Part model, mm, in its own coordinate system. A direction names the side the tool comes from. Give positions to 0.01 mm unless a question says otherwise; leave off trailing zeros. Order: outer loops, then holes, each group sorted by start corner. A loop starts at its lowest first (then second) coordinate and runs counter-clockwise, first axis right, second up.
1. Slice it at D-D on z = 10. List the corners of the cut face in (x, y).
2. Slice it at C-C on x = 0. Give the number of separate pieces and of enclosed holes in the cut face, and give its area (3 significant figures).
3. Drop flat-ended pins along their axis: pin 1 Ø10 at (x, z) = (6.5, -14.5) entering from -Y; pin 2 Ø12 at (x, y) = (42.5, 106.5) entering from -Z; pin 3 Ø1 at (x, y) = (24.5, 27) entering from +Z; pin 4 Ø1 at (x, z) = (-0.5, 14.5) entering from -Y. Give the stop position or say it passes through.
4. Which spindle directions (+Z, -Z, +X, -X, +Y, -Y) get a long thin tool onto all of the face, cutting with end or side? Do faces 4 (the flat face through (55, 110, 6)), 5 (the flat face through (-12, 12, 8)), 6 (the flat face through (0, 33, -40)), 7 (the flat face through (-5.9, 121.5, -43)), 8 (the flat face through (-5.9, 121.5, 3)). Say none if no direction does.
5. Probe line 1 (Y direction, x = 0, z = -32.5); line 2 (Y direction, x = 0, z = -25); line 3 (Y direction, x = 0, z = -17). List the from-to ranges inside material, lowest first.
6. Mould opens along X. For faces 1 (the flat face through (55, 110, -24)), 2 (the flat face through (-12, 12, -26)), 3 (the flat face through (25, 43, -9)) say: +X half, -X half, draft (parallel to the pull), parting line (faces both ways), or undercut.
7. Slice it at B-B on z = -20. List the corners of the cut face in (x, y), and give its area (3 significant figures).
8. Slice it at A-A on y = 0. List the corners of the cut face in (x, z).
from build123d import *

# Parameters (mm, degrees)
BOSS_EXTRUDE1_DEPTH      = 3
BOSS_EXTRUDE1_DEPTH_BACK = 43
SKETCH1_R                = 25
SKETCH1_R_2              = 12.5
BOSS_EXTRUDE2_DEPTH      = 18
SKETCH2_R                = 28
SKETCH2_R_2              = 16
BOSS_EXTRUDE3_DEPTH      = 35
BOSS_EXTRUDE4_DEPTH      = 31
CUT_EXTRUDE1_DEPTH       = 152.558569537
CUT_EXTRUDE1_DEPTH_BACK  = 152.558569537
SKETCH3_W                = 34
SKETCH3_H                = 83.380174096
SKETCH4_R                = 18
SKETCH4_R_2              = 7.5
BOSS_EXTRUDE5_DEPTH      = 24
BOSS_EXTRUDE6_DEPTH      = 21
BOSS_EXTRUDE7_DEPTH      = 9


with BuildPart() as part:
    # Sketch1 → Boss-Extrude1 (new, two sides: drawn at the far end of the back side and taken through both)
    with BuildSketch(Plane.XY.offset(-BOSS_EXTRUDE1_DEPTH_BACK)):
        with Locations((0, 110)):
            Circle(SKETCH1_R)
        with Locations((0, 110)):
            Circle(SKETCH1_R_2, mode=Mode.SUBTRACT)
    extrude(amount=BOSS_EXTRUDE1_DEPTH + BOSS_EXTRUDE1_DEPTH_BACK)

    # Sketch1_3 → Boss-Extrude2 (add)
    with BuildSketch(Plane.XY):
        with BuildLine():
            ThreePointArc((25, 110), (0, 85), (-25, 110))
            Line((-25, 110), (-25, 40))
            Line((-25, 40), (25, 40))
            Line((25, 40), (25, 110))
        make_face()
    extrude(amount=-BOSS_EXTRUDE2_DEPTH)



with BuildPart() as body_2:
    # Sketch2 → Boss-Extrude3 (new, symmetric)
    with BuildSketch(Plane.XY.offset(-9)):
        Circle(SKETCH2_R)
        Circle(SKETCH2_R_2, mode=Mode.SUBTRACT)
    extrude(amount=BOSS_EXTRUDE3_DEPTH, both=True)


with BuildPart() as part_1:
    add(part.part)

    add(body_2.part)  # Boss-Extrude4 merges body 2
    # Sketch2_3 → Boss-Extrude4 (add, symmetric)
    with BuildSketch(Plane.XY.offset(-9)):
        with BuildLine():
            Line((25, 40), (-25, 40))
            Line((-25, 40), (-25, 12.609520213))
            ThreePointArc((-25, 12.609520213), (0, 28), (25, 12.609520213))
            Line((25, 12.609520213), (25, 40))
        make_face()
    extrude(amount=BOSS_EXTRUDE4_DEPTH, both=True)

    # Sketch3 → Cut-Extrude1 (cut, two sides: drawn at the far end of the back side and taken through both)
    with BuildSketch(Plane.ZY.offset(25).offset(-CUT_EXTRUDE1_DEPTH_BACK)):
        with Locations((-9, -13.690087048)):
            Rectangle(SKETCH3_W, SKETCH3_H)
    extrude(amount=CUT_EXTRUDE1_DEPTH + CUT_EXTRUDE1_DEPTH_BACK, mode=Mode.SUBTRACT)



with BuildPart() as body_2_2:
    # Sketch4 → Boss-Extrude5 (new, symmetric)
    with BuildSketch(Plane.XY.offset(-9)):
        with Locations((85, 110)):
            Circle(SKETCH4_R)
        with Locations((85, 110)):
            Circle(SKETCH4_R_2, mode=Mode.SUBTRACT)
    extrude(amount=BOSS_EXTRUDE5_DEPTH, both=True)

    # Sketch4_3 → Boss-Extrude6 (add, symmetric)
    with BuildSketch(Plane.XY.offset(-9)):
        with BuildLine():
            Line((55, 110), (67, 110))
            ThreePointArc((67, 110), (72.272077939, 122.727922061), (85, 128))
            Line((85, 128), (55, 128))
            Line((55, 128), (55, 110))
        make_face()
        with BuildLine():
            ThreePointArc((85, 92), (72.272077939, 97.272077939), (67, 110))
            Line((67, 110), (55, 110))
            Line((55, 110), (55, 92))
            Line((55, 92), (85, 92))
        make_face()
    extrude(amount=BOSS_EXTRUDE6_DEPTH, both=True)


with BuildPart() as part_2:
    add(part_1.part)

    add(body_2_2.part)  # Boss-Extrude7 merges body 2 2
    # Sketch4_4 → Boss-Extrude7 (add, symmetric)
    with BuildSketch(Plane.XY.offset(-9)):
        with BuildLine():
            Line((25, 110), (55, 110))
            Line((55, 110), (55, 128))
            Line((55, 128), (17.349351573, 128))
            ThreePointArc((17.349351573, 128), (23.007974588, 119.779218033), (25, 110))
        make_face()
        with BuildLine():
            Line((55, 92), (55, 110))
            Line((55, 110), (25, 110))
            ThreePointArc((25, 110), (23.007974588, 100.220781967), (17.349351573, 92))
            Line((17.349351573, 92), (55, 92))
        make_face()
    extrude(amount=BOSS_EXTRUDE7_DEPTH, both=True)


solid = part_2.part
Data:
1. outline: (-25, 12.61) arc R28 ccw (long way) to (25, 12.61) - (25, 40) - (-25, 40) - close; (55, 92) - (85, 92) arc R18 ccw to (85, 128) - (55, 128) - close; hole circle Ø32 at (0, 0); hole circle Ø15 at (85, 110)
2. separate pieces: 4
2. enclosed holes: 0
2. area: 3,570 mm2
3. pin 1: stops at y = 28
3. pin 2: stops at z = -18
3. pin 3: stops at z = 22
3. pin 4: stops at y = -28
4. face 4: +Z, +Y, -Y
4. face 5: +X, -X, -Y
4. face 6: -Z
4. face 7: -Z, +X, -X, +Y
4. face 8: +Z, -X, +Y
5. line 1: y = -28 to -16, 16 to 40, 85 to 97.5, 122.5 to 135
5. line 2: y = 28 to 40, 85 to 97.5, 122.5 to 135
5. line 3: y = 28 to 97.5, 122.5 to 135
6. face 1: undercut
6. face 2: draft
6. face 3: +X half
7. outline: (-25, 28) - (25, 28) - (25, 40) - (-25, 40) - close; circle Ø50 at (0, 110); (55, 92) - (85, 92) arc R18 ccw to (85, 128) - (55, 128) - close; hole circle Ø25 at (0, 110); hole circle Ø15 at (85, 110)
7. area: 3,480 mm2
8. outline: (-28, -44) - (-16, -44) - (-16, -26) - (-28, -26) - close; (-28, 8) - (-16, 8) - (-16, 26) - (-28, 26) - close; (16, -44) - (28, -44) - (28, -26) - (16, -26) - close; (16, 8) - (28, 8) - (28, 26) - (16, 26) - close
